Read the model definition and answer for the solid it produces. Units are mm, in the model's axes. A direction names the side the tool comes from. Coordinates: 2 decimals unless noted, no trailing zeros. Order: outer loops, then holes, each group sorted by start corner. A loop starts at its lowest first (then second) coordinate and runs counter-clockwise, first axis right, second up. Notation, with made-up numbers: (44, -24) - (59, -24) arc R21 cw to (59, -20) - close; hole circle Ø8 at (19.5, 58.5). An arc over 180 degrees is marked (long way). Use one line per item in the form item = value.
Autodesk Inventor part; units mm, degrees
ref_plane "YZ Plane" through (0, 0, 0) normal (1, 0, 0) x (0, 1, 0)
ref_plane "XZ Plane" through (0, 0, 0) normal (0, 1, 0) x (-1, 0, 0)
ref_plane "XY Plane" through (0, 0, 0) normal (0, 0, 1) x (1, 0, 0)
sketch "Szkic1" plane through (0, 0, 0) normal (0, 1, 0) x (-1, 0, 0)
  circle A0 centre (0, 0) radius 2.5
  line L0 (0, 0) -> (0, -4)
  line L1 (0, 0) -> (0, 4)
  circle A1 centre (0, 0) radius 4
  line L2 (5.4643, 0) -> (-5.9483, 0)
  line L3 (0, 4) -> (2.5, 4)
  line L4 (0, 4) -> (-2.5, 4)
  line L5 (2.5, 4) -> (3.5955, 1.7528)
  line L6 (3.5955, 1.7528) -> (4.45, 0)
  line L7 (4.45, 0) -> (3.5955, -1.7528)
  line L8 (3.5955, -1.7528) -> (2.5, -4)
  line L9 (2.5, -4) -> (0, -4)
  line L10 (0, -4) -> (-2.5, -4)
  line L11 (-2.5, 4) -> (-3.5955, 1.7528)
  line L12 (-3.5955, 1.7528) -> (-4.45, 0)
  line L13 (-2.5, -4) -> (-4.45, 0)
  point P0 (-3.5955, -1.7528)
  dimension "d0" = 5
  dimension "d1" = 4
  dimension "d2" = 4
  dimension "d3" = 8
  dimension "d4" = 2.5
  dimension "d5" = 2.5
extrude "Wyciągnięcie proste2" add sketch "Szkic1" along normal blind 2.2 contours L2 L7 A1 | A1 L6 L2 | L3 L5 A1 | A1 L11 L4 | L10 L13 A1 | A1 L8 L9 | L2 L12 A1 | A1 L13 L2
extrude "Wyciągnięcie proste3" add sketch "Szkic1" along normal blind 2.45 contours L2 L1 A0 | L2 A1 L0 A0 | A0 L1 A1 L2 | A0 L0 L2 | L1 L2 A0 | A0 L2 A1 L1 | L0 A1 L2 A0 | A0 L2 L0
sketch "Szkic2" plane through (0, 2.45, 0) normal (0, 1, 0) x (1, 0, 0)
  point P0 (0, 0)
  point P1 (0, 0)
hole "Otwór1" at (0, 2.45, 0) at (0, 2.45, 0) direction (0, -1, 0) diameter 4.134 depth 14.2 tip angle 118
fillet "Zaokrąglenie1" radius 0.25 1 edges at (4, 2.45, 0)
properties part number "nakretka"
(1) The mould has two halves that part along Z. Classify faces 6 (the flat face through (2.21, 2.2, -3.54)), 7 (the cylindrical face through (1.26, 1.21, -1.64)), 8 (the flat face through (3.46, 1.08, -2.03)): +Z half, -Z half, draft (parallel to the pull), parting line (faces both ways), or undercut.
Answer list:
face_6 = draft
face_7 = undercut
face_8 = -Z half
(2) Straight lines are drawn through the part: L1, parallel to Z at x = 0, y = 1.7; L2, parallel to Y at x = -4, z = -0.5; L3, parallel to X at y = 1.55, z = -1. For each, find the intervals that lie inside material, in ascending order.
Answer list:
L1 = -4 to -2.07, 2.07 to 4
L2 = 0 to 2.2
L3 = -3.96 to -1.81, 1.81 to 3.96
(3) Which of the six approach directions +Z, -Z, +X, -X, +Y, -Y give full straight-line access (tool end or side, diameter ignored) to faces 1 (the flat face through (-4.2, 2.2, 0)), 2 (the flat face through (2.21, 2.2, 3.55)), 3 (the flat face through (-2.19, 2.2, -3.54)), 4 (the flat face through (4.2, 2.2, 0)), 5 (the flat face through (-2.19, 2.2, 3.55))?
Answer list:
face_1 = -X, +Y
face_2 = +Z, +X, +Y
face_3 = -Z, -X, +Y
face_4 = +X, +Y
face_5 = +Z, -X, +Y
(4) Section A-A, the plane y = 1.6 is taken. Write down the section's boundary in (x, z).
Answer list:
outline = (-4.45, 0) - (-3.6, -1.75) - (-2.5, -4) - (2.5, -4) - (4.45, 0) - (3.6, 1.75) - (2.5, 4) - (-2.5, 4) - (-3.6, 1.75) - close; hole circle Ø4.13 at (0, 0)
(5) Given pin 1 Ø1.5 at (x, z) = (1, -0.5) entering from +Y, flat-ended and moving along its own axis, determine where the tip first touches the part or whether it passes through.
Answer list:
pin_1 = through
